Part model, mm, in its own coordinate system. A direction names the side the tool comes from. Give positions to 0.01 mm unless a question says otherwise; leave off trailing zeros. Order: outer loops, then holes, each group sorted by start corner. A loop starts at its lowest first (then second) coordinate and runs counter-clockwise, first axis right, second up. Notation, with made-up numbers: (-9, 58) -> (4, 58) arc R20 cw to (4, 63) -> close; hole circle Ø6 at (18.5, -5). An arc over 180 degrees is marked (long way). Write item = value, one per line. Start each with the question number.
(1) Two-plate mould, pull along Y, no slides. Class faces 1 (the flat face through (27, -21.5, 1)), 2 (the flat face through (29, 18.5, 1)), 3 (the cylindrical face through (-4.9, -12.93, 1.48)): pulls with the +Y half, pulls with the -Y half, needs draft (parallel to the pull), parting line crosses it, or undercut.
(2) Saw through at D-D, the plane y = 12.5. List the corners of the cut face in (x, z), then the cut area to 3 significant figures.
(3) Saw through at A-A, the plane y = -9.5. List the corners of the cut face in (x, z).
(4) Probe line 1 along Y through (x, z) = (37, 1.65); line 2 along Y through (x, z) = (0.5, 0.85); line 3 along X through (y, z) = (-5.5, 2.2). List the from-to ranges inside material, lowest first. Write a range as from..to.
(5) Saw through at B-B, the plane x = -33.6. List the corners of the cut face in (y, z), then the cut area to 3 significant figures.
(6) Saw through at C-C, the plane z = 1.95. List the corners of the cut face in (x, y).
(7) Flat gauge pins, fed straight in: pin 1 (1.5 mm diameter, centred on y = -19.5, z = 1, fed in from -X); pin 2 (0.9 mm diameter, centred on x = 12, z = 2, fed in from -Y); pin 3 (0.9 mm diameter, centred on y = -20, z = 1, fed in from +X); pin 4 (10 mm diameter, centred on x = -33.6, y = 12.5, fed in from -Z). Where does each tip first touch, or does it go through?
(8) Which spindle directions (+Z, -Z, +X, -X, +Y, -Y) get a long thin tool onto all of the face, cutting with end or side? Do faces 4 (the flat face through (-5.5, -6, 1)), 5 (the flat face through (-7.5, 20, 1)), 6 (the flat face through (0, -18.5, 1)), 7 (the flat face through (-43, -18.5, 1)). Say none if no direction does.
from build123d import *

# Parameters (mm, degrees)
CROQUIS1_R              = 3.15
SALIENTE_EXTRUIR1_DEPTH = 3


with BuildPart() as part:
    # Croquis1 → Saliente-Extruir1 (new body)
    with BuildSketch(Plane.XY):
        Polygon((8.3, 21.5), (-7.5, 21.5), (-7.5, 18.5), (-50, 18.5), (-50, -18.5), (-34.9, -18.5), (-34.9, -21.5), (-19.1, -21.5), (-19.1, -18.5), (19.2, -18.5), (19.2, -21.5), (35, -21.5), (35, -18.5), (50, -18.5), (50, 18.5), (8.3, 18.5), align=None)
        with BuildLine():
            ThreePointArc((-5.5, 0.5), (-4.914213562, 1.914213562), (-3.5, 2.5))
            Line((-3.5, 2.5), (29.7, 2.5))
            ThreePointArc((29.7, 2.5), (31.114213562, 1.914213562), (31.7, 0.5))
            Line((31.7, 0.5), (31.7, -11.5))
            ThreePointArc((31.7, -11.5), (31.114213562, -12.914213562), (29.7, -13.5))
            Line((29.7, -13.5), (-3.5, -13.5))
            ThreePointArc((-3.5, -13.5), (-4.914213562, -12.914213562), (-5.5, -11.5))
            Line((-5.5, -11.5), (-5.5, 0.5))
        make_face(mode=Mode.SUBTRACT)
        with Locations((-33.6, 12.5)):
            Circle(CROQUIS1_R, mode=Mode.SUBTRACT)
        with Locations((37, 12.5)):
            Circle(CROQUIS1_R, mode=Mode.SUBTRACT)
    extrude(amount=SALIENTE_EXTRUIR1_DEPTH)


solid = part.part
Results list:
q1.face_1 = pulls with the -Y half
q1.face_2 = pulls with the +Y half
q1.face_3 = undercut
q2.outline = (-50, 0) -> (-36.75, 0) -> (-36.75, 3) -> (-50, 3) -> close; (-30.45, 0) -> (33.85, 0) -> (33.85, 3) -> (-30.45, 3) -> close; (40.15, 0) -> (50, 0) -> (50, 3) -> (40.15, 3) -> close
q2.area = 262 mm^2
q3.outline = (-50, 0) -> (-5.5, 0) -> (-5.5, 3) -> (-50, 3) -> close; (31.7, 0) -> (50, 0) -> (50, 3) -> (31.7, 3) -> close
q4.line_1 = -18.5..9.35, 15.65..18.5
q4.line_2 = -18.5..-13.5, 2.5..21.5
q4.line_3 = -50..-5.5, 31.7..50
q5.outline = (-21.5, 0) -> (9.35, 0) -> (9.35, 3) -> (-21.5, 3) -> close; (15.65, 0) -> (18.5, 0) -> (18.5, 3) -> (15.65, 3) -> close
q5.area = 101 mm^2
q6.outline = (-50, -18.5) -> (-34.9, -18.5) -> (-34.9, -21.5) -> (-19.1, -21.5) -> (-19.1, -18.5) -> (19.2, -18.5) -> (19.2, -21.5) -> (35, -21.5) -> (35, -18.5) -> (50, -18.5) -> (50, 18.5) -> (8.3, 18.5) -> (8.3, 21.5) -> (-7.5, 21.5) -> (-7.5, 18.5) -> (-50, 18.5) -> close; hole circle Ø6.3 at (-33.6, 12.5); hole (-5.5, -11.5) arc R2 ccw to (-3.5, -13.5) -> (29.7, -13.5) arc R2 ccw to (31.7, -11.5) -> (31.7, 0.5) arc R2 ccw to (29.7, 2.5) -> (-3.5, 2.5) arc R2 ccw to (-5.5, 0.5) -> close; hole circle Ø6.3 at (37, 12.5)
q7.pin_1 = -34.9
q7.pin_2 = -18.5
q7.pin_3 = 35
q7.pin_4 = 0
q8.face_4 = +Z, -Z
q8.face_5 = +Z, -Z, -X, +Y
q8.face_6 = +Z, -Z, -Y
q8.face_7 = +Z, -Z, -X, -Y
